Autodesk Inventor part; units mm, degrees
ref_plane "YZ Plane" through (0, 0, 0) normal (1, 0, 0) x (0, 1, 0)
ref_plane "XZ Plane" through (0, 0, 0) normal (0, 1, 0) x (-1, 0, 0)
ref_plane "XY Plane" through (0, 0, 0) normal (0, 0, 1) x (1, 0, 0)
sketch "Sketch1" plane through (0, 0, 0) normal (0, 1, 0) x (-1, 0, 0)
  line L0 (-17.3414, 16.8049) -> (-57.3414, 16.8049)
  line L1 (-57.3414, 16.8049) -> (-57.3414, -103.1951)
  line L2 (-57.3414, -103.1951) -> (-17.3414, -103.1951)
  line L3 (-17.3414, -103.1951) -> (-17.3414, 16.8049)
  line L4 (-24.8414, -10.6951) -> (-49.8414, -10.6951)
  line L5 (-49.8414, -10.6951) -> (-49.8414, -75.6951)
  line L6 (-49.8414, -75.6951) -> (-24.8414, -75.6951)
  line L7 (-24.8414, -75.6951) -> (-24.8414, -10.6951)
  circle A0 centre (-24.8414, -10.6951) radius 2.5
  circle A1 centre (-24.8414, -75.6951) radius 2.5
  circle A2 centre (-49.8414, -75.6951) radius 2.5
  circle A3 centre (-49.8414, -10.6951) radius 2.5
  point P0 (0, 0)
  dimension "d0" = 40
  dimension "d1" = 120
  dimension "d4" = 25
  dimension "d5" = 65
  dimension "d6" = 27.5
  dimension "d7" = 7.5
  dimension "d8" = 5
  dimension "d9" = 5
  dimension "d10" = 5
  dimension "d11" = 5
extrude "Extrusion1" add sketch "Sketch1" along normal blind 6 contours L3 L2 L1 L0 | L4 A0 L7 A1 L6 A2 L5 A3
properties part number "steeringmountplate"
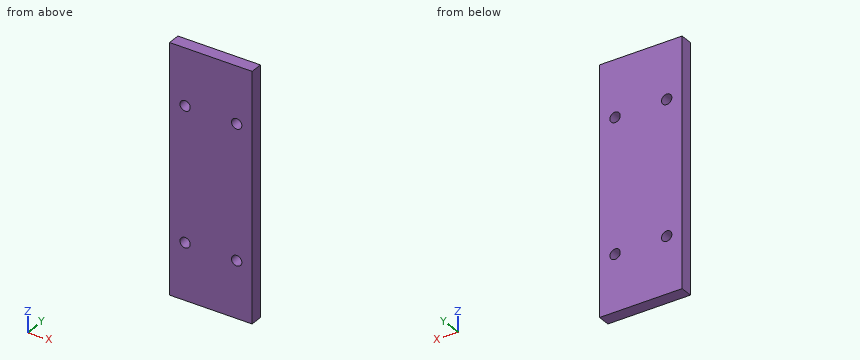
Design review of the part built by this model. Coordinates are the model's own, in mm. Coordinates: 2 decimals unless noted, no trailing zeros. Order: outer loops, then holes, each group sorted by start corner. A loop starts at its lowest first (then second) coordinate and runs counter-clockwise, first axis right, second up. Notation, with made-up numbers: (72, 15.5) -> (97, 15.5) arc R23 cw to (97, 43.5) -> close; hole circle Ø7 at (60.25, 31). An arc over 180 degrees is marked (long way). One line per item, written item: value.
1) We need section C-C, the plane x = 24. Give the boundary of the cut face in (y, z), then the cut area to 4 significant figures.
Output values:
outline: (0, -103.2) -> (6, -103.2) -> (6, -78.05) -> (0, -78.05) -> close; (0, -73.34) -> (6, -73.34) -> (6, -13.05) -> (0, -13.05) -> close; (0, -8.34) -> (6, -8.34) -> (6, 16.8) -> (0, 16.8) -> close
area: 663.5 mm2
2) We need section B-B, the plane y = 4.35. Give the boundary of the cut face in (x, z).
Output values:
outline: (17.34, -103.2) -> (57.34, -103.2) -> (57.34, 16.8) -> (17.34, 16.8) -> close; hole circle Ø5 at (24.84, -75.7); hole circle Ø5 at (24.84, -10.7); hole circle Ø5 at (49.84, -75.7); hole circle Ø5 at (49.84, -10.7)
3) To check wall thickness, follow probe 1 along Z at (x, y) = (50.5, 3.45); probe 2 along X at (y, z) = (3.8, -12.5). State the ranges of each line that lie inside material, in increasing order. Write a range as [from, to].
Output values:
probe 1: z = [-103.2, -78.11], [-73.28, -13.11], [-8.28, 16.8]
probe 2: x = [17.34, 23.11], [26.57, 48.11], [51.57, 57.34]
4) Clearance check with a flat-ended pin moving along its axis: P1, Ø6, axis at x = 24.84, z = -10.7, coming from the -Y side. State where the tip first meets the part, or that it passes through.
Output values:
P1: stops at y = 0
5) We need section A-A, the plane x = 48.5. Give the boundary of the cut face in (y, z).
Output values:
outline: (0, -103.2) -> (6, -103.2) -> (6, -77.8) -> (0, -77.8) -> close; (0, -73.59) -> (6, -73.59) -> (6, -12.8) -> (0, -12.8) -> close; (0, -8.59) -> (6, -8.59) -> (6, 16.8) -> (0, 16.8) -> close
